```python
from build123d import *

# Parameters (mm, degrees)
SALIENTE_EXTRUIR1_DEPTH = 3
SKETCH1_W               = 20
SKETCH1_H               = 7
SKETCH1_H_2             = 8
SKETCH1_W_2             = 7
SKETCH1_H_3             = 38.5
BOSS_EXTRUDE1_DEPTH     = 23
CUT_EXTRUDE1_DEPTH      = 85.65548432
SKETCH3_R               = 1.625
CUT_EXTRUDE2_DEPTH      = 73.427902257
CORTAR_EXTRUIR1_DEPTH   = 10
CORTAR_EXTRUIR2_REACH   = 71.098
CROQUIS4_R              = 1.25
CORTAR_EXTRUIR3_DEPTH   = 3
BOSS_EXTRUDE2_DEPTH     = 20
SALIENTE_EXTRUIR2_DEPTH = 59
CORTAR_EXTRUIR4_REACH   = 91.44
CROQUIS7_R              = 1.625
CORTAR_EXTRUIR5_START   = -2.42548
CORTAR_EXTRUIR5_DEPTH   = 4
SALIENTE_EXTRUIR4_START = -20
SALIENTE_EXTRUIR4_DEPTH = 20
CROQUIS17_W             = 7
CROQUIS17_H             = 23
CORTAR_EXTRUIR11_DEPTH  = 73.427902257
CUT_EXTRUDE3_DEPTH      = 85.65548432
LOCAL_FILES2_R          = 1.625
CUT_EXTRUDE4_DEPTH      = 10
CUT_EXTRUDE5_START      = -2.42548
CUT_EXTRUDE5_DEPTH      = 4


with BuildPart() as part:
    # Croquis1 → Saliente-Extruir1 (new body)
    with BuildSketch(Plane(origin=(0, 0, 0), x_dir=(1, 0, 0), z_dir=(0, 1, 0))):
        Polygon((-29.5, 32.640625), (29.5, 32.640625), (29.5, -47.359375), (8.5, -47.359375), (8.5, -27.453125), (3.5, -27.453125), (3.5, -47.359375), (-3.5, -47.359375), (-3.5, -27.453125), (-8.5, -27.453125), (-8.5, -47.359375), (-29.5, -47.359375), align=None)
    extrude(amount=SALIENTE_EXTRUIR1_DEPTH)

    # Sketch1 → Boss-Extrude1 (add)
    with BuildSketch(Plane(origin=(0, 3, 0), x_dir=(1, 0, 0), z_dir=(0, 1, 0))):
        with Locations((0, 19.640625)):
            Rectangle(SKETCH1_W, SKETCH1_H)
        with Locations((0, -12.359375)):
            Rectangle(SKETCH1_W, SKETCH1_H_2)
        with Locations((0, -35.609375)):
            Rectangle(SKETCH1_W_2, SKETCH1_H_3)
    extrude(amount=BOSS_EXTRUDE1_DEPTH)

    # Sketch2 → Cut-Extrude1 (cut, through all)
    with BuildSketch(Plane(origin=(29.5, 0, 0), x_dir=(0, 0, -1), z_dir=(1, 0, 0))):
        Polygon((-54.859375, 26), (-46.359375, 0), (-47.359375, 0), (-47.359375, 3), (-54.859375, 3), align=None)
    extrude(amount=-CUT_EXTRUDE1_DEPTH, mode=Mode.SUBTRACT)

    # Sketch3 → Cut-Extrude2 (cut, through all)
    with BuildSketch(Plane.ZY.offset(10)):
        with Locations((12.359375, 5.75)):
            Circle(SKETCH3_R)
        with Locations((12.359375, 23.25)):
            Circle(SKETCH3_R)
    extrude(amount=-CUT_EXTRUDE2_DEPTH, mode=Mode.SUBTRACT)

    # Croquis2 → Cortar-Extruir1 (cut)
    with BuildSketch(Plane(origin=(0, 0, -23.140625), x_dir=(-1, 0, 0), z_dir=(0, 0, -1))):
        Polygon((-5, 6), (-5, 3), (5, 3), (5, 6), (5, 21), (-5, 21), align=None)
    extrude(amount=-CORTAR_EXTRUIR1_DEPTH, mode=Mode.SUBTRACT)

    # Croquis3 → Cortar-Extruir2 (cut, up to next)
    with BuildSketch(Plane.ZY.offset(3.5), mode=Mode.PRIVATE) as cortar_extruir2_sk1:
        Polygon((21.90625, 3), (36.90625, 3), (36.90625, 26), (21.90625, 26), (16.359375, 26), (16.359375, 3), align=None)
    cortar_extruir2_tool1 = extrude(cortar_extruir2_sk1.sketch, amount=-CORTAR_EXTRUIR2_REACH, mode=Mode.PRIVATE) & part.part
    add(cortar_extruir2_tool1.solids().sort_by_distance((-3.5, 14.5, 26.632812))[0], mode=Mode.SUBTRACT)

    # Croquis4 → Cortar-Extruir3 (cut)
    with BuildSketch(Plane.XZ):
        with Locations(Location((-24.5, -22.640625, 0), (0, 0, 270))):
            Circle(CROQUIS4_R)
        with Locations(Location((-16.5, -22.640625, 0), (0, 0, 270))):
            Circle(CROQUIS4_R)
        with Locations(Location((-16.5, -12.640625, 0), (0, 0, 270))):
            Circle(CROQUIS4_R)
        with Locations(Location((-16.5, -2.640625, 0), (0, 0, 270))):
            Circle(CROQUIS4_R)
        with Locations(Location((-16.5, 7.359375, 0), (0, 0, 270))):
            Circle(CROQUIS4_R)
        with Locations(Location((-16.5, 17.359375, 0), (0, 0, 270))):
            Circle(CROQUIS4_R)
        with Locations(Location((-16.5, 27.359375, 0), (0, 0, 270))):
            Circle(CROQUIS4_R)
        with Locations(Location((-16.5, 37.359375, 0), (0, 0, 270))):
            Circle(CROQUIS4_R)
        with Locations(Location((-24.5, -12.640625, 0), (0, 0, 270))):
            Circle(CROQUIS4_R)
        with Locations(Location((-24.5, -2.640625, 0), (0, 0, 270))):
            Circle(CROQUIS4_R)
        with Locations(Location((-24.5, 7.359375, 0), (0, 0, 270))):
            Circle(CROQUIS4_R)
        with Locations(Location((-24.5, 17.359375, 0), (0, 0, 270))):
            Circle(CROQUIS4_R)
        with Locations(Location((-24.5, 27.359375, 0), (0, 0, 270))):
            Circle(CROQUIS4_R)
        with Locations(Location((-24.5, 37.359375, 0), (0, 0, 270))):
            Circle(CROQUIS4_R)
        with Locations(Location((16.5, 37.359375, 0), (0, 0, 270))):
            Circle(CROQUIS4_R)
        with Locations(Location((24.5, 37.359375, 0), (0, 0, 270))):
            Circle(CROQUIS4_R)
        with Locations(Location((16.5, 27.359375, 0), (0, 0, 270))):
            Circle(CROQUIS4_R)
        with Locations(Location((24.5, 27.359375, 0), (0, 0, 270))):
            Circle(CROQUIS4_R)
        with Locations(Location((16.5, 17.359375, 0), (0, 0, 270))):
            Circle(CROQUIS4_R)
        with Locations(Location((24.5, 17.359375, 0), (0, 0, 270))):
            Circle(CROQUIS4_R)
        with Locations(Location((24.5, 7.359375, 0), (0, 0, 270))):
            Circle(CROQUIS4_R)
        with Locations(Location((16.5, 7.359375, 0), (0, 0, 270))):
            Circle(CROQUIS4_R)
        with Locations(Location((16.5, -2.640625, 0), (0, 0, 270))):
            Circle(CROQUIS4_R)
        with Locations(Location((24.5, -2.640625, 0), (0, 0, 270))):
            Circle(CROQUIS4_R)
        with Locations(Location((24.5, -12.640625, 0), (0, 0, 270))):
            Circle(CROQUIS4_R)
        with Locations(Location((16.5, -12.640625, 0), (0, 0, 270))):
            Circle(CROQUIS4_R)
        with Locations(Location((16.5, -22.640625, 0), (0, 0, 270))):
            Circle(CROQUIS4_R)
        with Locations(Location((24.5, -22.640625, 0), (0, 0, 270))):
            Circle(CROQUIS4_R)
        with Locations(Location((6, 22.084531493, 0), (0, 0, 270))):
            Circle(CROQUIS4_R)
        with Locations(Location((-6, 22.084531493, 0), (0, 0, 270))):
            Circle(CROQUIS4_R)
        with Locations(Location((6, 2.359375, 0), (0, 0, 270))):
            Circle(CROQUIS4_R)
        with Locations(Location((-6, 2.359375, 0), (0, 0, 270))):
            Circle(CROQUIS4_R)
        with Locations(Location((-6, -7.640625, 0), (0, 0, 270))):
            Circle(CROQUIS4_R)
        with Locations(Location((6, -7.640625, 0), (0, 0, 270))):
            Circle(CROQUIS4_R)
    extrude(amount=-CORTAR_EXTRUIR3_DEPTH, mode=Mode.SUBTRACT)

    # Sketch5 → Boss-Extrude2 (add)
    with BuildSketch(Plane(origin=(-8.5, 0, 0), x_dir=(0, 0, -1), z_dir=(1, 0, 0))):
        Polygon((-36.90625, 3), (-36.90625, 0), (-46.359375, 0), (-47.340144231, 3), align=None)
    extrude(amount=BOSS_EXTRUDE2_DEPTH)

    # Croquis6 → Saliente-Extruir2 (add)
    with BuildSketch(Plane.ZY.offset(29.5)):
        Polygon((44.340144231, 3), (47.340144231, 3), (50.447532794, 12.504953252), (44.340144231, 14.501599513), (44.340144231, 6.347956044), align=None)
        Polygon((40.990144231, 3), (44.340144231, 3), (44.340144231, 6.347956044), align=None)
    extrude(amount=-SALIENTE_EXTRUIR2_DEPTH)

    # Cortar-Extruir4: up to this plane
    cortar_extruir4_end = Plane(origin=(29.5, 0, 44.340144231), z_dir=(0, 0, -1))
    # Croquis7 → Cortar-Extruir4 (cut, up to the surface)
    with BuildSketch(Plane(origin=(0, -13.692511694, 41.882976946), x_dir=(1, 0, 0), z_dir=(0, -0.31073885630742226, 0.9504953251756452)), mode=Mode.PRIVATE) as cortar_extruir4_sk1:
        with Locations(Location((-24.5, 22.561908251, 0), (0, 0, 270))):
            Circle(CROQUIS7_R)
    cortar_extruir4_tool1 = split(extrude(cortar_extruir4_sk1.sketch, amount=-CORTAR_EXTRUIR4_REACH, mode=Mode.PRIVATE), bisect_by=cortar_extruir4_end, keep=Keep.BOTH, mode=Mode.PRIVATE)
    add(cortar_extruir4_tool1.solids().sort_by_distance((-24.5, 7.752477, 48.893839))[0], mode=Mode.SUBTRACT)

    # Croquis8 → Cortar-Extruir5 (cut)
    with BuildSketch(Plane(origin=(0, -13.692511694, 41.882976946), x_dir=(1, 0, 0), z_dir=(0, -0.31073885630742226, 0.9504953251756452)).offset(CORTAR_EXTRUIR5_START)):
        Polygon((-22.91228676, 19.811908251), (-21.324573519, 22.561908251), (-22.91228676, 25.311908251), (-26.08771324, 25.311908251), (-27.675426481, 22.561908251), (-26.08771324, 19.811908251), align=None)
    extrude(amount=-CORTAR_EXTRUIR5_DEPTH, mode=Mode.SUBTRACT)

    # Croquis16 → Saliente-Extruir4 (add)
    with BuildSketch(Plane(origin=(10, 0, 0), x_dir=(0, 0, -1), z_dir=(1, 0, 0)).offset(SALIENTE_EXTRUIR4_START)):
        Polygon((-8.359375, 6), (-5.359375, 3), (-8.359375, 3), align=None)
        Polygon((-19.359375, 3), (-16.359375, 3), (-16.359375, 6), align=None)
    extrude(amount=SALIENTE_EXTRUIR4_DEPTH)

    # Croquis17 → Cortar-Extruir11 (cut, through all)
    with BuildSketch(Plane.ZY.offset(10)):
        with Locations((-19.640625, 14.5)):
            Rectangle(CROQUIS17_W, CROQUIS17_H)
    extrude(amount=-CORTAR_EXTRUIR11_DEPTH, mode=Mode.SUBTRACT)

    # Local Files1 → Cut-Extrude3 (cut, through all)
    with BuildSketch(Plane.ZY.offset(29.5)):
        Polygon((36.90625, 3), (40.990144231, 3), (44.340144231, 6.347956044), (44.340144231, 14.501599513), (50.447532794, 12.504953252), (54.859375, 26), (36.90625, 26), align=None)
    extrude(amount=-CUT_EXTRUDE3_DEPTH, mode=Mode.SUBTRACT)

    # Local Files2 → Cut-Extrude4 (cut)
    with BuildSketch(Plane(origin=(0, -13.692511694, 41.882976946), x_dir=(1, 0, 0), z_dir=(0, -0.31073885630742226, 0.9504953251756452))):
        with Locations(Location((0, 22.561908251, 0), (0, 0, 270))):
            Circle(LOCAL_FILES2_R)
        with Locations(Location((-24.5, 22.561908251, 0), (0, 0, 270))):
            Circle(LOCAL_FILES2_R)
        with Locations(Location((24.5, 22.561908251, 0), (0, 0, 270))):
            Circle(LOCAL_FILES2_R)
    extrude(amount=-CUT_EXTRUDE4_DEPTH, mode=Mode.SUBTRACT)

    # Local Files4 → Cut-Extrude5 (cut)
    with BuildSketch(Plane(origin=(0, -13.692511694, 41.882976946), x_dir=(1, 0, 0), z_dir=(0, -0.31073885630742226, 0.9504953251756452)).offset(CUT_EXTRUDE5_START)):
        Polygon((1.58771324, 19.811908251), (3.175426481, 22.561908251), (1.58771324, 25.311908251), (-1.58771324, 25.311908251), (-3.175426481, 22.561908251), (-1.58771324, 19.811908251), align=None)
        Polygon((26.08771324, 19.811908251), (27.675426481, 22.561908251), (26.08771324, 25.311908251), (22.91228676, 25.311908251), (21.324573519, 22.561908251), (22.91228676, 19.811908251), align=None)
    extrude(amount=-CUT_EXTRUDE5_DEPTH, mode=Mode.SUBTRACT)


solid = part.part
```
For this review, take the finished solid that the model builds, in its own axes (mm). A direction names the side the tool comes from. Round coordinates to 2 decimals unless told otherwise and drop trailing zeros. Write each loop counter-clockwise with the first axis right and the second up, starting at its lowest first coordinate (ties: lowest second). Pieces come first, ordered by that corner, then holes. Notation, with made-up numbers: M 55,62 L 111,62 A11 cw 111,66 Z; hole C -3,16 d8. An arc over 180 degrees is marked long. One line per item, written item: value. Start each with the question number.
(1) We need section D-D (z = 4.5). Give the boundary of the cut face in (x, y).
(2) Wall thickness on line 1 (X direction, y = 2, z = -22); line 2 (X direction, y = 11.25, z = 11.5); line 3 (Y direction, x = -17, z = -6.5): over which ranges is each line inside the solid? List them lowest first.
(3) Machinability: for faces 1 (the flat face through (25.87, 9.7, 46.98)), 2 (the flat face through (24.52, 11.62, 45.91)), 3 (the flat face through (-3.5, 1, 32)), 4 (the flat face through (-0.41, 4.7, 42.69)), which of the approach directions +Z, -Z, +X, -X, +Y, -Y give a long, thin tool a straight path to every point of the face, cutting with its end or side? Answer none if there is none.
(4) We need section A-A (x = -6). Count the separate pieces of the cut face and the enclosed holes in it, and give its area (3 significant figures).
(5) The part is to be moulded in two halves that separate along Z. For faces 5 (the flat face through (3.5, 1, 32)), 6 (the flat face through (-29.5, 1, 15)), 7 (the flat face through (-0.4, 13.5, 47.4)), say which applies: released by +Z, released by -Z, zero draft, split by the parting line, or undercut.
(6) We need section C-C (x = -13.5). Give the boundary of the cut face in (y, z).
(7) We need section B-B (y = 23.25). Give the boundary of the cut face in (x, z).
(8) Insertion check: pin 1 (2 mm diameter, centred on x = 10.5, y = 9.5, fed in from +Z); pin 2 (3 mm diameter, centred on x = -15, y = 7, fed in from +Z); pin 3 (6 mm diameter, centred on x = -2, y = 14.5, fed in from -Z). Each pin has a flat end and moves straight along its axis. Give the tip position at first contact, or say it passes through.
Result:
1. outline: M -29.5,0 L 29.5,0 L 29.5,3 L -29.5,3 Z
2. line 1: -29.5 to -25.57, -23.43 to -17.57, -15.43 to 15.43, 17.57 to 23.43, 25.57 to 29.5
2. line 2: -10 to 10
2. line 3: 0 to 3
3. face 1: none
3. face 2: -Z
3. face 3: +Y, -Y
3. face 4: +X, -X, +Y
4. separate pieces: 5
4. enclosed holes: 2
4. area: 419 mm²
5. face 5: undercut
5. face 6: zero draft
5. face 7: released by +Z
6. outline: M 0,-32.64 L 3,-32.64 L 3,40.99 L 6.35,44.34 L 14.5,44.34 L 12.5,50.45 L 0,46.36 Z
7. outline: M -10,8.36 L 10,8.36 L 10,10.73 L -10,10.73 Z; M -10,13.98 L 10,13.98 L 10,16.36 L -10,16.36 Z
8. pin 1: z = 49.79
8. pin 2: z = 49.14
8. pin 3: z = 8.36
